Source: CAD feature listing. Evaluate the final solid. Frame: model axes, mm. Round coordinates to 2 decimals unless told otherwise and drop trailing zeros. Loops run counter-clockwise (first coordinate to the right, second up) from the corner with the lowest first, then second, coordinate; pieces in that order, holes last.
Item 1: Section query A-A on z = 1.3. Return loops of the section in (x, y).
Item 2: First-contact query: P1, Ø3.5, axis at x = -20.53, y = -10.67, coming from the +Z side; P2, Ø5, axis at x = -88.53, y = -15.67, coming from the +Z side; P3, Ø2.5, axis at x = -30.53, y = -10.67, coming from the +Z side. Flat tips, straight axial feed; report the tip coordinate or a pass-through.
Item 3: Ray query, L1, parallel to X at y = -20.5, z = 1.65; L2, parallel to X at y = -10.5, z = 1.4; L3, parallel to Y at x = -22.5, z = 0.7. Return the intervals inside material, ascending.
Autodesk Inventor part; units mm, degrees
ref_plane "YZ Plane" through (0, 0, 0) normal (1, 0, 0) x (0, 1, 0)
ref_plane "XZ Plane" through (0, 0, 0) normal (0, 1, 0) x (-1, 0, 0)
ref_plane "XY Plane" through (0, 0, 0) normal (0, 0, 1) x (1, 0, 0)
sketch "Эскиз1" plane through (0, 0, 0) normal (0, 0, 1) x (1, 0, 0)
  circle A0 centre (37.4694, -15.6747) radius 1.5
  circle A1 centre (-20.5306, -10.6747) radius 1.5
  circle A2 centre (-20.5306, -20.6747) radius 1.5
  arc A3 (37.4694, -25.6747) -> (42.4694, -20.6747) centre (37.4694, -20.6747) ccw
  line L0 (42.4694, -10.6747) -> (42.4694, -20.6747)
  arc A4 (42.4694, -10.6747) -> (37.4694, -5.6747) centre (37.4694, -10.6747) ccw
  line L1 (-25.5306, -5.6747) -> (37.4694, -5.6747)
  line L2 (-25.5306, -25.6747) -> (-25.5306, -5.6747)
  line L3 (37.4694, -25.6747) -> (-25.5306, -25.6747)
  arc A5 (42.3694, -10.6747) -> (37.4694, -5.7747) centre (37.4694, -10.6747) ccw
  line L4 (42.3694, -10.6747) -> (42.3694, -20.6747)
  arc A6 (37.4694, -25.5747) -> (42.3694, -20.6747) centre (37.4694, -20.6747) ccw
  line L5 (37.4694, -25.5747) -> (-25.5306, -25.5747)
  line L6 (-25.5306, -5.7747) -> (37.4694, -5.7747)
  point P0 (0, 0)
  dimension "d0" = 0.1
extrude "Выдавливание1" add sketch "Эскиз1" along normal blind 2 contours L2 L6 A5 L4 A6 L5
chamfer "Фаска1" distance 2 angle 45 3 edges at (35.9694, -15.6747, 2) (-22.0306, -20.6747, 2) (-22.0306, -10.6747, 2)
mirror "Зеркальное отражение1" about plane through (-25.5306, -5.7747, 0) normal (-1, 0, 0)
properties part number "РеброСкрепления"
Data:
1. outline: (-93.43, -20.67) arc R4.9 ccw to (-88.53, -25.57) - (37.47, -25.57) arc R4.9 ccw to (42.37, -20.67) - (42.37, -10.67) arc R4.9 ccw to (37.47, -5.77) - (-88.53, -5.77) arc R4.9 ccw to (-93.43, -10.67) - close; hole circle Ø5.6 at (-88.53, -15.67); hole circle Ø5.6 at (-30.53, -20.67); hole circle Ø5.6 at (-30.53, -10.67); hole circle Ø5.6 at (-20.53, -20.67); hole circle Ø5.6 at (-20.53, -10.67); hole circle Ø5.6 at (37.47, -15.67)
2. P1: stops at z = 0.26
2. P2: stops at z = 1.01
2. P3: passes through
3. L1: x = -93.43 to -33.68, -27.39 to -23.68, -17.39 to 42.37
3. L2: x = -93.43 to -33.42, -27.64 to -23.42, -17.64 to 42.37
3. L3: y = -25.57 to -21.65, -19.7 to -11.65, -9.7 to -5.77
